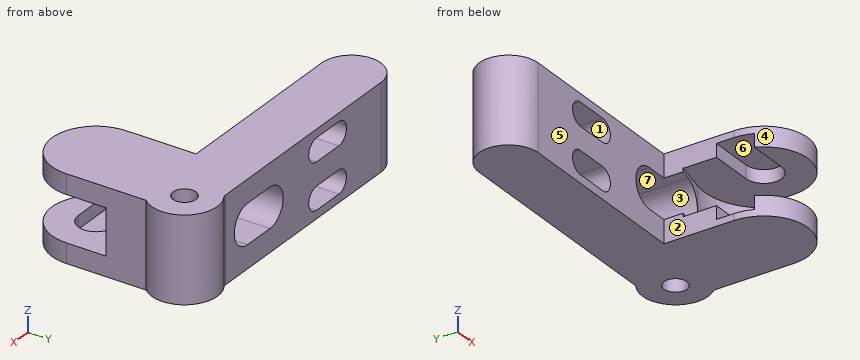
Autodesk Inventor part; units mm, degrees
ref_plane "YZ Plane" through (0, 0, 0) normal (1, 0, 0) x (0, 1, 0)
ref_plane "XZ Plane" through (0, 0, 0) normal (0, 1, 0) x (-1, 0, 0)
ref_plane "XY Plane" through (0, 0, 0) normal (0, 0, 1) x (1, 0, 0)
sketch "Sketch1" plane through (0, 0, 0) normal (0, 0, 1) x (1, 0, 0)
  circle A0 centre (0, 0) radius 2.7
  line L0 (0, 0) -> (0, 13) construction
  line L1 (-6.7, 0) -> (-6.7, 13)
  line L2 (6.7, 13) -> (6.7, 0)
  arc A1 (-6.7, 0) -> (6.7, 0) centre (0, 0) ccw
  arc A2 (6.7, 13) -> (-6.7, 13) centre (0, 13) ccw
  circle A3 centre (0, 0) radius 2.5 construction
  line L3 (-35, 15.2) -> (0, 15.2) construction
  line L4 (-35, 10.7) -> (0, 10.7)
  line L5 (0, 19.7) -> (-35, 19.7)
  arc A4 (-35, 19.7) -> (-35, 10.7) centre (-35, 15.2) ccw
  arc A5 (0, 10.7) -> (0, 19.7) centre (0, 15.2) ccw
  line L6 (0, 13) -> (0, 19.7) construction
  circle A6 centre (3, 15.5) radius 1.5 construction
  circle A7 centre (3, 15.5) radius 5
  point P0 (0, 6.5)
  point P1 (-17.5, 15.2)
  dimension "d2" = 0.2
  dimension "d3" = 4
  dimension "d5" = 13
  dimension "d10" = 9
  dimension "d11" = 35
  dimension "d12" = 10
extrude "Extrusion1" add sketch "Sketch1" along normal blind 13
sketch "Sketch8" plane through (0, 0, 13) normal (0, 0, 1) x (1, 0, 0)
  line L0 (0, 2.7) -> (-16.9826, 2.7)
  line L1 (-16.9826, -2.7) -> (0, -2.7)
  arc A0 (0, -2.7) -> (0, 2.7) centre (0, 0) ccw
  arc A1 (-16.9826, 2.7) -> (-16.9826, -2.7) centre (-16.9826, 0) ccw
  circle A2 centre (0, 0) radius 2.7 construction
  line L2 (-16.9826, 0) -> (0, 0) construction
  point P0 (-3.3627, 0)
  dimension "d25" = 16.9826
extrude "Extrusion6" cut sketch "Sketch8" against normal through all
sketch "Sketch9" plane through (0, 0, 13) normal (0, 0, 1) x (1, 0, 0)
  arc A0 (0, -2.7) -> (0, 2.7) centre (0, 0) ccw construction
  arc A1 (-6.1319, -2.7) -> (6.7, 0) centre (0, 0) ccw construction
  line L0 (0, 0) -> (0, 13) construction
  line L1 (6.7, 0) -> (6.7, 13)
  line L2 (-6.7, 13) -> (-6.7, 0)
  arc A2 (-6.7, 0) -> (6.7, 0) centre (0, 0) ccw
  arc A3 (6.7, 13) -> (-6.7, 13) centre (0, 13) ccw construction
  line L3 (0, 19.7) -> (-35, 19.7)
  line L4 (-6.7, 13) -> (6.7, 13)
  point P0 (0, 6.5)
extrude "Extrusion7" add sketch "Sketch9" against normal blind 1
ref_plane "Work Plane1" through (0, 0, 6.5) normal (0, 0, 1) x (1, 0, 0)
mirror "Mirror3" about plane through (0, 0, 6.5) normal (0, 0, 1) of "Extrusion7"
sketch "Sketch2" plane through (-35, 19.7, 0) normal (0, 1, 0) x (1, 0, 0)
  circle A0 centre (12, -3) radius 1.6 construction
  line L0 (52.5, -6.5) -> (-14, -6.5) construction
  line L1 (9.5, -3) -> (14.5, -3) construction
  line L2 (9.5, -4.75) -> (14.5, -4.75)
  line L3 (14.5, -1.25) -> (9.5, -1.25)
  arc A1 (9.5, -1.25) -> (9.5, -4.75) centre (9.5, -3) ccw
  arc A2 (14.5, -4.75) -> (14.5, -1.25) centre (14.5, -3) ccw
  point P0 (35, 0)
  dimension "d6" = 3.5
  dimension "d7" = 5
extrude "Extrusion2" cut sketch "Sketch2" against normal through all
ref_plane "Work Plane2" through (0, 0, 0) normal (1, 0, 0) x (0, 0, -1)
sketch "Sketch4" plane through (0, 0, 0) normal (1, 0, 0) x (0, 0, -1)
  line L0 (-4, -7.79) -> (-4, 7.79) construction
  line L1 (-8.79, -8) -> (-4.21, -8) construction
  line L2 (-9, -7.79) -> (-9, 7.79) construction
  line L3 (-8.79, 8) -> (-4.21, 8) construction
  line L4 (-4.21, 8) -> (-4, 8) construction
  line L5 (-4, 8) -> (-4, 7.79) construction
  line L6 (-9, -7.79) -> (-9, -8) construction
  line L7 (-9, -8) -> (-8.79, -8) construction
  line L8 (-4, 8) -> (-9, -8) construction
  line L9 (-10, -9) -> (-3, -9)
  line L10 (-3, -9) -> (-3, 9)
  line L11 (-3, 9) -> (-10, 9)
  line L12 (-10, 9) -> (-10, -9)
  line L13 (0, 0) -> (-13, 0)
  line L14 (-10, -9) -> (-3, 9) construction
  line L15 (-3, -9) -> (-10, 9) construction
  line L16 (-3, 0) -> (-10, 0)
  point P0 (-6.5, 0)
  dimension "d15" = 1
  dimension "d16" = 1
revolve "Revolution1" cut sketch "Sketch4" angle 360 about axis through (0, 0, 0) along (0, 0, 1) contours L12 L13 L10 L9
sketch "Sketch5" plane through (0, 0, 13) normal (0, 0, 1) x (1, 0, 0)
  arc A0 (6.7, 12.137) -> (0.2781, 19.6942) centre (3, 15.5) ccw construction
  circle A1 centre (3, 15.5) radius 1.75
  point P0 (0, 0)
  dimension "d18" = 3.5
extrude "Extrusion3" cut sketch "Sketch5" against normal through all
sketch "Sketch7" plane through (0, 0, 3) normal (0, 0, 1) x (0.9786, 0.2059, 0)
  line L0 (0, 0) -> (0, 9) construction
  arc A0 (7.7937, 4.5008) -> (-5.3191, 7.26) centre (0, 0) ccw construction
  line L1 (-6.7, -9) -> (6.7, -9)
  line L2 (6.7, -9) -> (6.7, 9)
  line L3 (6.7, 9) -> (-6.7, 9)
  line L4 (-6.7, 9) -> (-6.7, -9)
  line L5 (-6.7, -9) -> (6.7, 9) construction
  line L6 (6.7, -9) -> (-6.7, 9) construction
  line L7 (7.7937, 4.5008) -> (6.5564, -1.3796) construction
  line L8 (-6.7, -9) -> (0, -9)
  line L9 (0, -9) -> (0, 9)
  line L10 (0, 9) -> (-6.7, 9)
  line L11 (-6.7, 9) -> (-6.7, -9)
extrude "Extrusion5" cut sketch "Sketch7" along normal up to surface (7 mm away) contours L4 L3 L9 L1
mirror "Mirror4" about plane through (0, 0, 6.5) normal (0, 0, 1) of "Extrusion2"
sketch "Sketch10" plane through (-35, 19.7, 0) normal (0, 1, 0) x (1, 0, 0)
  circle A0 centre (27.5, -6.5) radius 4.35 construction
  line L0 (25, -6.5) -> (30, -6.5) construction
  line L1 (28.3, -3) -> (28.3, -10)
  line L2 (25, -9.5) -> (30, -9.5)
  line L3 (30, -3.5) -> (25, -3.5)
  arc A1 (25, -3.5) -> (25, -9.5) centre (25, -6.5) ccw
  arc A2 (30, -9.5) -> (30, -3.5) centre (30, -6.5) ccw
  point P0 (35, 0)
  dimension "d30" = 5
  dimension "d31" = 3
extrude "Extrusion8" cut sketch "Sketch10" against normal through all
properties part number "Extruder Clamp"
Input: part model. Units: mm. Frame: model coordinates. Face numbers are marked on the shaded views. A direction names the side the tool comes from. Round coordinates to 2 decimals unless told otherwise and drop trailing zeros. Write each loop counter-clockwise with the first axis right and the second up, starting at its lowest first coordinate (ties: lowest second). Pieces come first, ordered by that corner, then holes.
1) Reachability of the marked faces 5, 6 and 7 from +Z, -Z, +X, -X, +Y, -Y: full face, straight path, thin tool, end or side. Return the list, or none.
2) Cut plane C-C (y = 4.5). Return the cut outline in (x, z), then the cut area to 3 significant figures.
3) Contact query for flat-ended pins moving along their axis: P1, Ø6.5, axis at x = -14.5, z = 8.5, coming from the +Y side; P2, Ø1.5, axis at y = 3, z = 3, coming from the +X side; P3, Ø3, axis at x = -7.5, z = 10, coming from the -Y side. Output: stop coordinate, or through.
4) Ray query, L1, parallel to Z at x = -20.5, y = 16.75; L2, parallel to Z at x = -2.5, y = 0.75; L3, parallel to X at y = 11.75, z = 9.25. Return the intervals inside material, ascending.
5) Draft query along X for the marked faces 1, 2, 3 and 4. Return one class per face: pulls with the +X half, pulls with the -X half, needs draft (parallel to the pull), parting line crosses it, or undercut.
6) Cut plane D-D (x = 3.5). Return the cut outline in (y, z).
7) Cut plane B-B (y = 15). Return the cut outline in (x, z).
8) Cut plane A-A (z = 4). Return the cut outline in (x, y).
Geometry says:
1. face 5: +Z, -Z, -X, -Y
1. face 6: -X
1. face 7: +Y, -Y
2. outline: (-6.7, 0) - (6.7, 0) - (6.7, 3) - (-6.7, 3) - close; (-6.7, 10) - (6.7, 10) - (6.7, 13) - (-6.7, 13) - close
2. area: 80.4 mm2
3. P1: stops at y = 19.7
3. P2: stops at x = 6.7
3. P3: stops at y = -2.98
4. L1: z = 0 to 1.25, 4.75 to 8.25, 11.75 to 13
4. L2: z = 0 to 1, 12 to 13
4. L3: x = -37.89 to -27.08, -18.92 to -11.2, -3.8 to 6.7
5. face 1: undercut
5. face 2: pulls with the -X half
5. face 3: undercut
5. face 4: parting line crosses it
6. outline: (-5.71, 0) - (13.82, 0) - (13.82, 13) - (-5.71, 13) - (-5.71, 10) - (8.29, 10) - (8.29, 3) - (-5.71, 3) - close; (17.18, 0) - (20.47, 0) - (20.47, 13) - (17.18, 13) - close
7. outline: (-39.5, 0) - (1.32, 0) - (1.32, 13) - (-39.5, 13) - close; (4.68, 0) - (7.97, 0) - (7.97, 13) - (4.68, 13) - close; hole (-25.5, 1.25) - (-20.5, 1.25) arc R1.75 ccw to (-20.5, 4.75) - (-25.5, 4.75) arc R1.75 ccw to start; hole (-25.5, 8.25) - (-20.5, 8.25) arc R1.75 ccw to (-20.5, 11.75) - (-25.5, 11.75) arc R1.75 ccw to start; hole (-10, 3.5) - (-5, 3.5) arc R3 ccw to (-5, 9.5) - (-10, 9.5) arc R3 ccw to start
8. outline: (-35, 10.7) - (-26.94, 10.7) - (-26.94, 19.7) - (-35, 19.7) arc R4.5 ccw to start; (-19.06, 10.7) - (-11.66, 10.7) - (-11.66, 19.7) - (-19.06, 19.7) - close; (-3.34, 8.49) - (-1.85, 8.81) arc R9 cw to (6.7, 6.01) - (6.7, 12.14) arc R5 ccw to (0.28, 19.69) arc R6.7 ccw to (0, 19.7) - (-3.34, 19.7) - close; hole circle Ø3.5 at (3, 15.5)
